```python
from build123d import *

# Parameters (mm, degrees)
SKETCH_1_W           = 58
SKETCH_1_H           = 30
EXTRUDE_1_DEPTH      = 4
SKETCH_2_W           = 4
SKETCH_2_H           = 3
SKETCH_2_H_2         = 6
SKETCH_2_H_3         = 4
CUT_EXTRUDE_2_DEPTH  = 3
SKETCH_3_W           = 4
SKETCH_3_H           = 3
SKETCH_3_H_2         = 6
SKETCH_3_H_3         = 4
CUT_EXTRUDE_3_DEPTH  = 3
CUT_EXTRUDE_4_DEPTH  = 5
SKETCH_5_R           = 7.5
CUT_EXTRUDE_5_DEPTH  = 5
SKETCH_11_W          = 16
SKETCH_11_H          = 16
CUT_EXTRUDE_10_DEPTH = 10
SKETCH_12_W          = 40
SKETCH_12_H          = 5
EXTRUDE_2_DEPTH      = 4
SKETCH_13_R          = 2.5
EXTRUDE_3_DEPTH      = 2.5
SKETCH_14_R          = 1.1
CUT_EXTRUDE_11_DEPTH = 7.5
SKETCH_15_W          = 6.5
SKETCH_15_H          = 25
SKETCH_15_R          = 1.25
EXTRUDE_4_DEPTH      = 4
SKETCH_16_W          = 6.5
SKETCH_16_H          = 12.5
SKETCH_16_R          = 1.25
EXTRUDE_5_DEPTH      = 5
CUT_EXTRUDE_12_DEPTH = 5
FILLET_1_R           = 10
FILLET_2_R           = 5


with BuildPart() as part:
    # 草图1 → 凸台-拉伸1 (new body)
    with BuildSketch(Plane.XY):
        Rectangle(SKETCH_1_W, SKETCH_1_H)
    extrude(amount=EXTRUDE_1_DEPTH)

    # 草图2 → 切除-拉伸2 (cut)
    with BuildSketch(Plane(origin=(29, 0, 0), x_dir=(0, 0, -1), z_dir=(1, 0, 0))):
        with Locations((-2, 13.5)):
            Rectangle(SKETCH_2_W, SKETCH_2_H)
        with Locations((-2, 5)):
            Rectangle(SKETCH_2_W, SKETCH_2_H_2)
        with Locations((-2, 0)):
            Rectangle(SKETCH_2_W, SKETCH_2_H_3)
        with Locations((-2, -5)):
            Rectangle(SKETCH_2_W, SKETCH_2_H_2)
        with Locations((-2, -13.5)):
            Rectangle(SKETCH_2_W, SKETCH_2_H)
    extrude(amount=-CUT_EXTRUDE_2_DEPTH, mode=Mode.SUBTRACT)

    # 草图3 → 切除-拉伸3 (cut)
    with BuildSketch(Plane.ZY.offset(29)):
        with Locations((2, 13.5)):
            Rectangle(SKETCH_3_W, SKETCH_3_H)
        with Locations((2, 5)):
            Rectangle(SKETCH_3_W, SKETCH_3_H_2)
        with Locations((2, 0)):
            Rectangle(SKETCH_3_W, SKETCH_3_H_3)
        with Locations((2, -5)):
            Rectangle(SKETCH_3_W, SKETCH_3_H_2)
        with Locations((2, -13.5)):
            Rectangle(SKETCH_3_W, SKETCH_3_H)
    extrude(amount=-CUT_EXTRUDE_3_DEPTH, mode=Mode.SUBTRACT)

    # 草图4 → 切除-拉伸4 (cut, through all)
    with BuildSketch(Plane(origin=(0, 0, 0), x_dir=(-1, 0, 0), z_dir=(0, 0, -1))):
        Polygon((-26, 2), (-23.5, 2), (-23.5, 4), (-21, 4), (-21, -4), (-23.5, -4), (-23.5, -2), (-26, -2), align=None)
        Polygon((26, -2), (23.5, -2), (23.5, -4), (21, -4), (21, 4), (23.5, 4), (23.5, 2), (26, 2), align=None)
    extrude(amount=-CUT_EXTRUDE_4_DEPTH, mode=Mode.SUBTRACT)

    # 草图5 → 切除-拉伸5 (cut, through all)
    with BuildSketch(Plane(origin=(0, 0, 0), x_dir=(-1, 0, 0), z_dir=(0, 0, -1))):
        Circle(SKETCH_5_R)
        with BuildLine():
            Line((-9, 2.5), (9, 2.5))
            ThreePointArc((9, 2.5), (11.5, 0), (9, -2.5))
            Line((9, -2.5), (-9, -2.5))
            ThreePointArc((-9, -2.5), (-11.5, 0), (-9, 2.5))
        make_face()
    extrude(amount=-CUT_EXTRUDE_5_DEPTH, mode=Mode.SUBTRACT)

    # 草图11 → 切除-拉伸10 (cut)
    with BuildSketch(Plane.XY.offset(4)):
        Rectangle(SKETCH_11_W, SKETCH_11_H)
    extrude(amount=-CUT_EXTRUDE_10_DEPTH, mode=Mode.SUBTRACT)

    # 草图12 → 凸台-拉伸2 (add)
    with BuildSketch(Plane(origin=(0, 0, 0), x_dir=(-1, 0, 0), z_dir=(0, 0, -1))):
        with Locations((0, 17.5)):
            Rectangle(SKETCH_12_W, SKETCH_12_H)
        with Locations((0, -17.5)):
            Rectangle(SKETCH_12_W, SKETCH_12_H)
    extrude(amount=-EXTRUDE_2_DEPTH)

    # 草图13 → 凸台-拉伸3 (add)
    with BuildSketch(Plane(origin=(0, 0, 0), x_dir=(-1, 0, 0), z_dir=(0, 0, -1))):
        with Locations((14, -14)):
            Circle(SKETCH_13_R)
        with Locations((-14, -14)):
            Circle(SKETCH_13_R)
        with Locations((14, 14)):
            Circle(SKETCH_13_R)
        with Locations((-14, 14)):
            Circle(SKETCH_13_R)
    extrude(amount=EXTRUDE_3_DEPTH)

    # 草图14 → 切除-拉伸11 (cut, through all)
    with BuildSketch(Plane(origin=(0, 0, -2.5), x_dir=(-1, 0, 0), z_dir=(0, 0, -1))):
        with Locations((14, -14)):
            Circle(SKETCH_14_R)
        with Locations((-14, -14)):
            Circle(SKETCH_14_R)
        with Locations((-14, 14)):
            Circle(SKETCH_14_R)
        with Locations((14, 14)):
            Circle(SKETCH_14_R)
    extrude(amount=-CUT_EXTRUDE_11_DEPTH, mode=Mode.SUBTRACT)

    # 草图15 → 凸台-拉伸4 (add)
    with BuildSketch(Plane(origin=(0, 0, 0), x_dir=(-1, 0, 0), z_dir=(0, 0, -1))):
        with Locations((16.75, -32.5)):
            Rectangle(SKETCH_15_W, SKETCH_15_H)
        with Locations((15.5, -40)):
            Circle(SKETCH_15_R, mode=Mode.SUBTRACT)
        with Locations((-16.75, -32.5)):
            Rectangle(SKETCH_15_W, SKETCH_15_H)
        with Locations((-15.5, -40)):
            Circle(SKETCH_15_R, mode=Mode.SUBTRACT)
    extrude(amount=-EXTRUDE_4_DEPTH)

    # 草图16 → 凸台-拉伸5 (add)
    with BuildSketch(Plane(origin=(0, 0, 0), x_dir=(-1, 0, 0), z_dir=(0, 0, -1))):
        with Locations((16.75, -38.75)):
            Rectangle(SKETCH_16_W, SKETCH_16_H)
        with Locations((15.5, -40)):
            Circle(SKETCH_16_R, mode=Mode.SUBTRACT)
        with Locations((-16.75, -38.75)):
            Rectangle(SKETCH_16_W, SKETCH_16_H)
        with Locations((-15.5, -40)):
            Circle(SKETCH_16_R, mode=Mode.SUBTRACT)
    extrude(amount=EXTRUDE_5_DEPTH)

    # 草图17 → 切除-拉伸12 (cut, through all)
    with BuildSketch(Plane(origin=(0, 0, 0), x_dir=(-1, 0, 0), z_dir=(0, 0, -1))):
        Polygon((13.5, -20), (0, -15), (-13.5, -20), align=None)
    extrude(amount=-CUT_EXTRUDE_12_DEPTH, mode=Mode.SUBTRACT)

    # 圆角1
    fillet_1_edges = [part.edges().sort_by_distance(p)[0] for p in [
        (0, -15, 2),
    ]]
    fillet(fillet_1_edges, radius=FILLET_1_R)

    # 圆角2
    fillet_2_edges = [part.edges().sort_by_distance(p)[0] for p in [
        (13.5, -20, 2),
        (-13.5, -20, 2),
    ]]
    fillet(fillet_2_edges, radius=FILLET_2_R)


solid = part.part
```
Design review of the part built by this model. Coordinates are the model's own, in mm. A direction names the side the tool comes from. Give positions to 0.01 mm unless a question says otherwise; leave off trailing zeros. Loops run counter-clockwise (first coordinate to the right, second up) from the corner with the lowest first, then second, coordinate; pieces in that order, holes last. Notation, with made-up numbers: M 79.25,56.25 L 137.25,56.25 A23 ccw 137.25,90.25 Z; hole C -12.5,89 d8. An arc over 180 degrees is marked long. Return JSON: item names as keys, results as strings. Group by question number.
Item 1: We need section A-A (z = -3.25). Give the boundary of the cut face in (x, y).
Item 2: We need section C-C (x = 5.5). Give the boundary of the cut face in (y, z), and give its area (3 significant figures).
Item 3: Tool access review of faces 1 (the flat face through (0, 8, 2)), 2 (the flat face through (20, -34, 0)), 3 (the flat face through (-20, -34, 1)), 4 (the flat face through (-26, 5, 2)): name each direction out of +Z, -Z, +X, -X, +Y, -Y from which nothing blocks a thin tool from reaching the whole face with its end or side.
Item 4: We need section B-B (y = 14). Give the boundary of the cut face in (x, z).
Item 5: Mouldability with a two-part tool opening along Y and no side actions: class faces 5 (the flat face through (21, 0, 2)), 6 (the flat face through (0, 20, 2)), 7 (the flat face through (29, 10, 2)) as released by +Y, released by -Y, zero draft, split by the parting line, or undercut.
Item 6: We need section D-D (y = -40). Give the boundary of the cut face in (x, z), and give its area (3 significant figures).
Item 7: For probe 1 along Y at (x, z) = (14, 0.5); probe 2 along X at (y, z) = (-3, 1); probe 3 along Y at (x, z) = (15.5, 1.35), list the stretches that pass through material, from the lowest coordinate up.
Item 8: Insertion check: pin 1 Ø2 at (x, z) = (25.5, 2) entering from -Y; pin 2 Ø2.5 at (x, y) = (-14, 14) entering from -Z; pin 3 Ø3 at (y, z) = (-21, -2) entering from +X; pin 4 Ø6 at (x, y) = (15.5, -21) entering from -Z. Each pin has a flat end and moves straight along its axis. Give the tip position at first contact, or say it passes through.
Output:
{
 "1": {"outline": "M -20,-45 L -13.5,-45 L -13.5,-32.5 L -20,-32.5 Z; M 13.5,-45 L 20,-45 L 20,-32.5 L 13.5,-32.5 Z; hole C -15.5,-40 d2.5; hole C 15.5,-40 d2.5"},
 "2": {"outline": "M -17.04,0 L -8,0 L -8,4 L -17.04,4 Z; M 8,0 L 20,0 L 20,4 L 8,4 Z", "area": "84.1 mm^2"},
 "3": {"face 1": "+Z, -Z", "face 2": "+Z, -Z, +X, -Y", "face 3": "+Z, -Z, -X, -Y", "face 4": "+Z, -Z, -X"},
 "4": {"outline": "M -26,0 L -16.5,0 L -16.5,-2.5 L -15.1,-2.5 L -15.1,4 L -26,4 Z; M -12.9,-2.5 L -11.5,-2.5 L -11.5,0 L 11.5,0 L 11.5,-2.5 L 12.9,-2.5 L 12.9,4 L -12.9,4 Z; M 15.1,-2.5 L 16.5,-2.5 L 16.5,0 L 26,0 L 26,4 L 15.1,4 Z"},
 "5": {"face 5": "undercut", "face 6": "released by +Y", "face 7": "zero draft"},
 "6": {"outline": "M -20,-5 L -16.75,-5 L -16.75,4 L -20,4 Z; M -14.25,-5 L -13.5,-5 L -13.5,4 L -14.25,4 Z; M 13.5,-5 L 14.25,-5 L 14.25,4 L 13.5,4 Z; M 16.75,-5 L 20,-5 L 20,4 L 16.75,4 Z", "area": "72.0 mm^2"},
 "7": {"probe 1": "y = -45 to -15.1, -12.9 to 12.9, 15.1 to 20", "probe 2": "x = -26 to -23.5, -21 to -8, 8 to 21, 23.5 to 26", "probe 3": "y = -45 to -41.25, -38.75 to 20"},
 "8": {"pin 1": "stops at y = -15", "pin 2": "stops at z = -2.5", "pin 3": "passes through", "pin 4": "stops at z = 0"}
}
